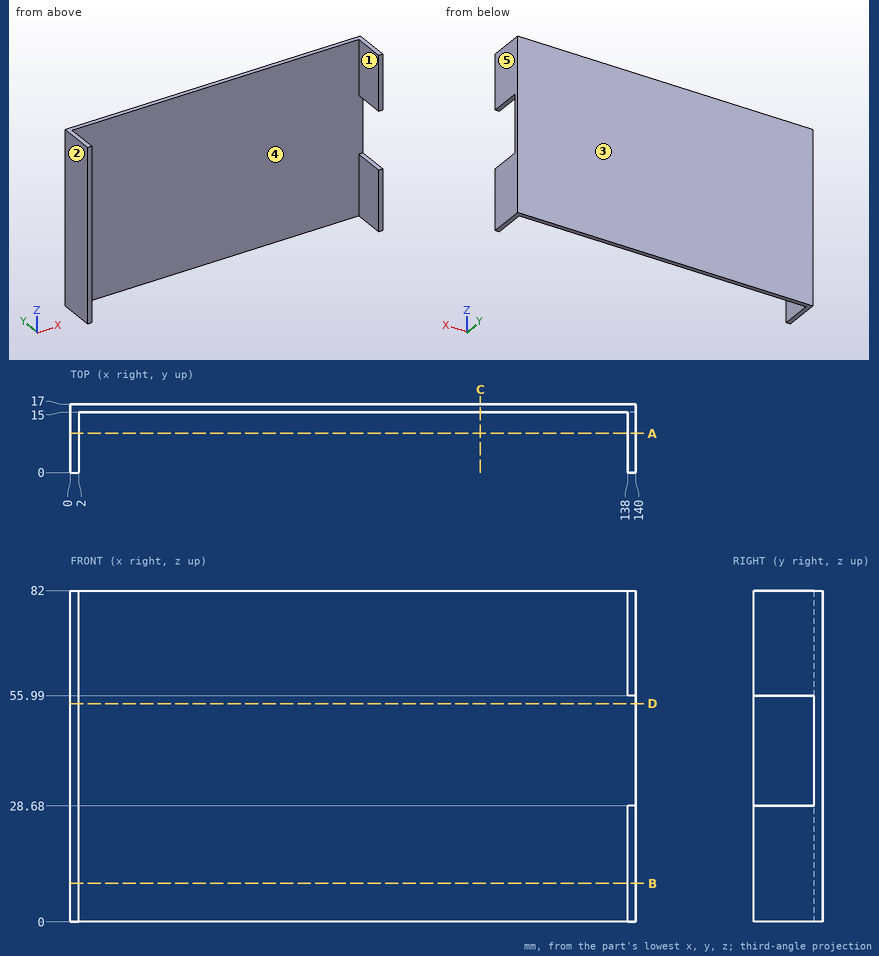
The figure shows three views and two pictorial views of one solid part (mm, origin at its lowest corner). Answer the questions. A direction names the side the tool comes from. Round coordinates to 2 decimals unless told otherwise and drop trailing zeros. Loops run counter-clockwise (first coordinate to the right, second up) from the corner with the lowest first, then second, coordinate; pieces in that order, holes last. Notation, with made-up numbers: (84, -23.75) -> (101, -23.75) arc R9 ccw to (101, -19.75) -> close; hole circle Ø10 at (19, 24.25). An arc over 180 degrees is marked (long way). Use one line per item in the form item = value.
(1) Straight lines are drawn through the part: line 1 (X direction, y = 7.75, z = 68); line 2 (X direction, y = 4, z = 46.5); line 3 (Y direction, x = 82.5, z = 38). For each, find the intervals that lie inside material, in ascending order.
Answer list:
line_1 = 0 to 2, 138 to 140
line_2 = 0 to 2
line_3 = 15 to 17
(2) Find section A-A on y = 9.75. Give the vertices of the cut face in (x, z), then the cut area to 3 significant figures.
Answer list:
outline = (0, 0) -> (2, 0) -> (2, 82) -> (0, 82) -> close; (138, 0) -> (140, 0) -> (140, 28.68) -> (138, 28.68) -> close; (138, 55.99) -> (140, 55.99) -> (140, 82) -> (138, 82) -> close
area = 273 mm2
(3) Find section C-C on x = 101.5. Give the vertices of the cut face in (y, z), then the cut area to 3 significant figures.
Answer list:
outline = (15, 0) -> (17, 0) -> (17, 82) -> (15, 82) -> close
area = 164 mm2
(4) Find section B-B on z = 9.5. Give the vertices of the cut face in (x, y), then the cut area to 3 significant figures.
Answer list:
outline = (0, 0) -> (2, 0) -> (2, 15) -> (138, 15) -> (138, 0) -> (140, 0) -> (140, 17) -> (0, 17) -> close
area = 340 mm2
(5) Find section D-D on z = 54. Give the vertices of the cut face in (x, y).
Answer list:
outline = (0, 0) -> (2, 0) -> (2, 15) -> (140, 15) -> (140, 17) -> (0, 17) -> close
(6) A flat-ended cylindrical pin translates along its axis: P1, Ø10, axis at x = 84.5, y = 12, coming from the +Z side. Find the tip coordinate at first contact, or state that the pin passes through.
Answer list:
P1 = 82
(7) A tool of negligible diameter and unlimited length cuts with its end or side. For the marked faces 1 and 2, from which of +Z, -Z, +X, -X, +Y, -Y can it reach the whole face along a straight path? Write none if from no direction.
Answer list:
face_1 = +Z, -Z, -Y
face_2 = +Z, -Z, -X, +Y, -Y
(8) For a pull along X with two mould halves and no side action, classify the marked faces 3, 4 and 5 as released by +X, released by -X, zero draft, split by the parting line, or undercut.
Answer list:
face_3 = zero draft
face_4 = undercut
face_5 = released by +X
